Read the model definition and answer for the solid it produces. Units are mm, in the model's axes. Face numbers are marked on the shaded views. A direction names the side the tool comes from. Round coordinates to 2 decimals unless told otherwise and drop trailing zeros. Order: outer loops, then holes, each group sorted by start corner. A loop starts at its lowest first (then second) coordinate and runs counter-clockwise, first axis right, second up. Notation, with made-up numbers: (42.5, 49.25) -> (73.5, 49.25) arc R24 ccw to (73.5, 70.25) -> close; hole circle Ø6 at (78, 61). An arc over 180 degrees is marked (long way). Answer as a JSON object with one key per item and string values. Group by question number.
Item 1: Section B-B, the plane z = 8 is taken. Write down the section's boundary in (x, y).
Item 2: Section D-D, the plane z = 33.6 is taken. Write down the section's boundary in (x, y), plus the area to 3 significant figures.
Item 3: Given P1, Ø5, axis at x = 0.5, y = 17.5, coming from the +Z side; P2, Ø1.5, axis at x = 0.5, y = 19, coming from the -Z side; P3, Ø5, axis at x = 10, y = 10, coming from the -Z side, each flat-ended and moving along its own axis, determine where each tip first touches the part or whether it passes through.
Item 4: For the marked faces 4, 5, 6, 7 and 8, determine the directions among +Z, -Z, +X, -X, +Y, -Y from which every point of the face is accessible in a straight line to the end or side of a thin tool.
Item 5: Section C-C, the plane y = 5.75 is taken. Write down the section's boundary in (x, z).
Item 6: Consider probe 1 along Y at (x, z) = (-15.5, 43.4); probe 2 along Y at (x, z) = (15.5, 43.3); probe 3 along Z at (x, y) = (-19, -15). Determine where each line is inside the solid, lowest interval first. Write a range as from..to.
Item 7: The mould has two halves that part along Z. Classify the marked faces 1, 2 and 3: pulls with the +Z half, pulls with the -Z half, needs draft (parallel to the pull), parting line crosses it, or undercut.
Item 8: Section A-A, the plane z = -6 is taken. Count the separate pieces of the cut face and the enclosed holes in it, plus the area to 3 significant figures.
from build123d import *

# Parameters (mm, degrees)
SKETCH1_W               = 46
SKETCH1_H               = 47
BOSS_EXTRUDE1_DEPTH     = 9
SKETCH3_W               = 46
SKETCH3_H               = 10
BOSS_EXTRUDE2_DEPTH     = 11
BOSS_EXTRUDE5_DEPTH     = 15
SKETCH8_W               = 7
SKETCH8_H               = 2
CUT_EXTRUDE3_DEPTH      = 24
CUT_EXTRUDE3_DEPTH_BACK = 24
SKETCH11_W              = 46
SKETCH11_H              = 8
BOSS_EXTRUDE6_DEPTH     = 34
SKETCH12_W              = 46
SKETCH12_H              = 58.5
BOSS_EXTRUDE7_DEPTH     = 1
CUT_EXTRUDE6_REACH      = 57
SKETCH13_R              = 15
SKETCH13_R_2            = 1.6
SKETCH14_W              = 46
SKETCH14_H              = 5
BOSS_EXTRUDE8_DEPTH     = 11.5
SKETCH15_W              = 16
SKETCH15_H              = 15.996045694
CUT_EXTRUDE7_DEPTH      = 3
SKETCH2_R               = 1.6
CUT_EXTRUDE1_DEPTH      = 36
CUT_EXTRUDE1_DEPTH_BACK = 21
SKETCH9_R               = 3.5
CUT_EXTRUDE4_DEPTH      = 2
FILLET1_R               = 3
SKETCH17_R              = 1.5
CUT_EXTRUDE8_DEPTH      = 47
SKETCH20_R              = 1.5
CUT_EXTRUDE10_DEPTH     = 10


with BuildPart() as part:
    # Sketch1 → Boss-Extrude1 (new body)
    with BuildSketch(Plane.XY):
        Rectangle(SKETCH1_W, SKETCH1_H)
    extrude(amount=BOSS_EXTRUDE1_DEPTH)

    # Sketch3 → Boss-Extrude2 (add)
    with BuildSketch(Plane.XY):
        with Locations((0, 18.5)):
            Rectangle(SKETCH3_W, SKETCH3_H)
        with Locations((0, -18.5)):
            Rectangle(SKETCH3_W, SKETCH3_H)
    extrude(amount=-BOSS_EXTRUDE2_DEPTH)

    # Sketch7 → Boss-Extrude5 (add)
    with BuildSketch(Plane(origin=(0, 0, -11), x_dir=(-1, 0, 0), z_dir=(0, 0, -1))):
        Polygon((-23, 23.5), (-11, 23.5), (-11, 25.5), (-17, 28.044850705), (-23, 25.5), align=None)
        Polygon((17, 28.044850705), (11, 25.5), (11, 23.5), (23, 23.5), (23, 25.5), align=None)
    extrude(amount=-BOSS_EXTRUDE5_DEPTH)

    # Sketch8 → Cut-Extrude3 (cut, two sides)
    with BuildSketch(Plane(origin=(0, 0, 0), x_dir=(0, 0, -1), z_dir=(1, 0, 0))) as cut_extrude3_sk:
        with Locations((3.5, 24.5)):
            Rectangle(SKETCH8_W, SKETCH8_H)
    extrude(amount=CUT_EXTRUDE3_DEPTH, mode=Mode.SUBTRACT)
    extrude(cut_extrude3_sk.sketch, amount=-CUT_EXTRUDE3_DEPTH_BACK, mode=Mode.SUBTRACT)

    # Sketch11 → Boss-Extrude6 (add)
    with BuildSketch(Plane.XY.offset(9)):
        with Locations((0, -19.5)):
            Rectangle(SKETCH11_W, SKETCH11_H)
        with Locations((0, 31)):
            Rectangle(SKETCH11_W, SKETCH11_H)
    extrude(amount=BOSS_EXTRUDE6_DEPTH)

    # Sketch12 → Boss-Extrude7 (add)
    with BuildSketch(Plane.XY.offset(43)):
        with Locations((0, 5.75)):
            Rectangle(SKETCH12_W, SKETCH12_H)
    extrude(amount=BOSS_EXTRUDE7_DEPTH)

    # Sketch13 → Cut-Extrude6 (cut, up to next)
    with BuildSketch(Plane.XY.offset(44), mode=Mode.PRIVATE) as cut_extrude6_sk1:
        with Locations((0, 5.75)):
            Circle(SKETCH13_R)
    cut_extrude6_tool1 = extrude(cut_extrude6_sk1.sketch, amount=-CUT_EXTRUDE6_REACH, mode=Mode.PRIVATE) & part.part
    add(cut_extrude6_tool1.solids().sort_by_distance((0, 5.75, 44))[0], mode=Mode.SUBTRACT)
    # Sketch13 → Cut-Extrude6 (cut, up to next)
    with BuildSketch(Plane.XY.offset(44), mode=Mode.PRIVATE) as cut_extrude6_sk2:
        with Locations((-15.5, 21.25)):
            Circle(SKETCH13_R_2)
    cut_extrude6_tool2 = extrude(cut_extrude6_sk2.sketch, amount=-CUT_EXTRUDE6_REACH, mode=Mode.PRIVATE) & part.part
    add(cut_extrude6_tool2.solids().sort_by_distance((-15.5, 21.25, 44))[0], mode=Mode.SUBTRACT)
    # Sketch13 → Cut-Extrude6 (cut, up to next)
    with BuildSketch(Plane.XY.offset(44), mode=Mode.PRIVATE) as cut_extrude6_sk3:
        with Locations((15.5, 21.25)):
            Circle(SKETCH13_R_2)
    cut_extrude6_tool3 = extrude(cut_extrude6_sk3.sketch, amount=-CUT_EXTRUDE6_REACH, mode=Mode.PRIVATE) & part.part
    add(cut_extrude6_tool3.solids().sort_by_distance((15.5, 21.25, 44))[0], mode=Mode.SUBTRACT)
    # Sketch13 → Cut-Extrude6 (cut, up to next)
    with BuildSketch(Plane.XY.offset(44), mode=Mode.PRIVATE) as cut_extrude6_sk4:
        with Locations((15.5, -9.75)):
            Circle(SKETCH13_R_2)
    cut_extrude6_tool4 = extrude(cut_extrude6_sk4.sketch, amount=-CUT_EXTRUDE6_REACH, mode=Mode.PRIVATE) & part.part
    add(cut_extrude6_tool4.solids().sort_by_distance((15.5, -9.75, 44))[0], mode=Mode.SUBTRACT)
    # Sketch13 → Cut-Extrude6 (cut, up to next)
    with BuildSketch(Plane.XY.offset(44), mode=Mode.PRIVATE) as cut_extrude6_sk5:
        with Locations((-15.5, -9.75)):
            Circle(SKETCH13_R_2)
    cut_extrude6_tool5 = extrude(cut_extrude6_sk5.sketch, amount=-CUT_EXTRUDE6_REACH, mode=Mode.PRIVATE) & part.part
    add(cut_extrude6_tool5.solids().sort_by_distance((-15.5, -9.75, 44))[0], mode=Mode.SUBTRACT)

    # Sketch14 → Boss-Extrude8 (add)
    with BuildSketch(Plane(origin=(0, 23.5, 0), x_dir=(1, 0, 0), z_dir=(0, 1, 0))):
        with Locations((0, -6.5)):
            Rectangle(SKETCH14_W, SKETCH14_H)
    extrude(amount=BOSS_EXTRUDE8_DEPTH)

    # Sketch15 → Cut-Extrude7 (cut)
    with BuildSketch(Plane.XY.offset(44)):
        with Locations((15, 5.75)):
            Rectangle(SKETCH15_W, SKETCH15_H)
    extrude(amount=-CUT_EXTRUDE7_DEPTH, mode=Mode.SUBTRACT)

    # Sketch2 → Cut-Extrude1 (cut, two sides)
    with BuildSketch(Plane.XY.offset(9)) as cut_extrude1_sk:
        with Locations((-10, 10)):
            Circle(SKETCH2_R)
        with Locations((10, 10)):
            Circle(SKETCH2_R)
        with Locations((-10, -10)):
            Circle(SKETCH2_R)
        with Locations((10, -10)):
            Circle(SKETCH2_R)
    extrude(amount=CUT_EXTRUDE1_DEPTH, mode=Mode.SUBTRACT)
    extrude(cut_extrude1_sk.sketch, amount=-CUT_EXTRUDE1_DEPTH_BACK, mode=Mode.SUBTRACT)

    # Sketch9 → Cut-Extrude4 (cut)
    with BuildSketch(Plane.XY.offset(9)):
        with Locations((-10, 10)):
            Circle(SKETCH9_R)
        with Locations((10, 10)):
            Circle(SKETCH9_R)
        with Locations((10, -10)):
            Circle(SKETCH9_R)
        with Locations((-10, -10)):
            Circle(SKETCH9_R)
    extrude(amount=-CUT_EXTRUDE4_DEPTH, mode=Mode.SUBTRACT)

    # Fillet1
    fillet1_edges = [part.edges().sort_by_distance(p)[0] for p in [
        (20, 26.772425352, 4),
        (14, 26.772425352, 4),
        (11, 24.5, 4),
        (-20, 26.772425352, 4),
        (-11, 24.5, 4),
        (-14, 26.772425352, 4),
        (0, 23.5, 4),
    ]]
    fillet(fillet1_edges, radius=FILLET1_R)

    # Sketch17 → Cut-Extrude8 (cut, through all)
    with BuildSketch(Plane.ZY.offset(23)):
        with Locations((40, -19.5)):
            Circle(SKETCH17_R)
        with Locations((33.6, -19.5)):
            Circle(SKETCH17_R)
        with Locations((27.2, -19.5)):
            Circle(SKETCH17_R)
        with Locations((20.8, -19.5)):
            Circle(SKETCH17_R)
        with Locations((14.4, -19.5)):
            Circle(SKETCH17_R)
        with Locations((8, -19.5)):
            Circle(SKETCH17_R)
        with Locations((33.6, 31)):
            Circle(SKETCH17_R)
        with Locations((27.2, 31)):
            Circle(SKETCH17_R)
        with Locations((20.8, 31)):
            Circle(SKETCH17_R)
        with Locations((14.4, 31)):
            Circle(SKETCH17_R)
        with Locations((8, 31)):
            Circle(SKETCH17_R)
        with Locations((40, 31)):
            Circle(SKETCH17_R)
    extrude(amount=-CUT_EXTRUDE8_DEPTH, mode=Mode.SUBTRACT)

    # Sketch20 → Cut-Extrude10 (cut)
    with BuildSketch(Plane(origin=(0, 0, -11), x_dir=(-1, 0, 0), z_dir=(0, 0, -1))):
        with Locations((-19, -18.5)):
            Circle(SKETCH20_R)
        with Locations((-12.666666667, -18.5)):
            Circle(SKETCH20_R)
        with Locations((-6.333333333, -18.5)):
            Circle(SKETCH20_R)
        with Locations((0, -18.5)):
            Circle(SKETCH20_R)
        with Locations((6.333333333, -18.5)):
            Circle(SKETCH20_R)
        with Locations((12.666666667, -18.5)):
            Circle(SKETCH20_R)
        with Locations((19, -18.5)):
            Circle(SKETCH20_R)
        with Locations((-19, 18.5)):
            Circle(SKETCH20_R)
        with Locations((-12.666666667, 18.5)):
            Circle(SKETCH20_R)
        with Locations((-6.333333333, 18.5)):
            Circle(SKETCH20_R)
        with Locations((0, 18.5)):
            Circle(SKETCH20_R)
        with Locations((6.333333333, 18.5)):
            Circle(SKETCH20_R)
        with Locations((12.666666667, 18.5)):
            Circle(SKETCH20_R)
        with Locations((19, 18.5)):
            Circle(SKETCH20_R)
    extrude(amount=-CUT_EXTRUDE10_DEPTH, mode=Mode.SUBTRACT)


solid = part.part
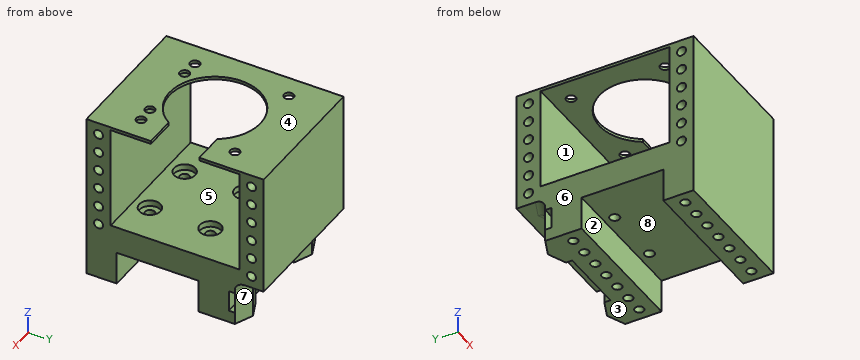
Values found:
{
 "1": {"outline": "(-23, -23.5) -> (23, -23.5) -> (23, -21) -> (-23, -21) -> close; (-23, -18) -> (23, -18) -> (23, 29.5) -> (-23, 29.5) -> close; (-23, 32.5) -> (23, 32.5) -> (23, 35) -> (-23, 35) -> close; hole circle Ø7 at (-10, -10); hole circle Ø7 at (-10, 10); hole circle Ø7 at (10, -10); hole circle Ø7 at (10, 10)"},
 "2": {"outline": "(-23, -23.5) -> (23, -23.5) -> (23, -21) -> (-23, -21) -> close; (-23, -18) -> (23, -18) -> (23, -15.5) -> (-23, -15.5) -> close; (-23, 27) -> (23, 27) -> (23, 29.5) -> (-23, 29.5) -> close; (-23, 32.5) -> (23, 32.5) -> (23, 35) -> (-23, 35) -> close", "area": "460 mm2"},
 "3": {"P1": "z = 9", "P2": "z = -1", "P3": "z = 0"},
 "4": {"face 4": "+Z, +X, -X, +Y, -Y", "face 5": "+X, -X", "face 6": "+Z, -Z, -X, +Y, -Y", "face 7": "-Z, +X, +Y", "face 8": "-Z, +X, -X"},
 "5": {"outline": "(-23, 0) -> (23, 0) -> (23, 9) -> (-23, 9) -> close; (-23, 43) -> (-15, 43) -> (-15, 44) -> (-23, 44) -> close"},
 "6": {"probe 1": "-23.5..-11.35, -8.15..19.65, 22.85..35", "probe 2": "-23.5..-11.35, -8.15..-2.25, 13.75..19.65, 22.85..35", "probe 3": "-11..9, 43..44"},
 "7": {"face 1": "undercut", "face 2": "needs draft", "face 3": "pulls with the -Z half"},
 "8": {"separate pieces": "4", "enclosed holes": "14", "area": "852 mm2"}
}
